```python
from build123d import *

# Parameters (mm, degrees)
EXTRUDE_1_DEPTH     = 15
SKETCH_2_R          = 1.25
CUT_EXTRUDE_1_DEPTH = 30.154759474
SKETCH_3_R          = 1.25
CUT_EXTRUDE_2_DEPTH = 30.154759474
SKETCH_4_R          = 1.5
CUT_EXTRUDE_3_DEPTH = 18
SKETCH_5_W          = 25
SKETCH_5_H          = 15
CUT_EXTRUDE_4_DEPTH = 1
SKETCH_6_W          = 25
SKETCH_6_H          = 15
CUT_EXTRUDE_5_DEPTH = 1


with BuildPart() as part:
    # 草图1 → 凸台-拉伸1 (new body)
    with BuildSketch(Plane(origin=(0, 0, 0), x_dir=(1, 0, 0), z_dir=(0, 1, 0))):
        Polygon((0, 0), (-5, 0), (-5, -15), (20, -15), (20, 0), (15, 0), (15, -11), (0, -11), align=None)
    extrude(amount=EXTRUDE_1_DEPTH)

    # 草图2 → 切除-拉伸1 (cut, through all)
    with BuildSketch(Plane(origin=(0, 0, 0), x_dir=(-1, 0, 0), z_dir=(0, 0, -1))):
        with Locations((-17.5, 4)):
            Circle(SKETCH_2_R)
        with Locations((-17.5, 11)):
            Circle(SKETCH_2_R)
    extrude(amount=-CUT_EXTRUDE_1_DEPTH, mode=Mode.SUBTRACT)

    # 草图3 → 切除-拉伸2 (cut, through all)
    with BuildSketch(Plane(origin=(0, 0, 0), x_dir=(-1, 0, 0), z_dir=(0, 0, -1))):
        with Locations((2.5, 4)):
            Circle(SKETCH_3_R)
        with Locations((2.5, 11)):
            Circle(SKETCH_3_R)
    extrude(amount=-CUT_EXTRUDE_2_DEPTH, mode=Mode.SUBTRACT)

    # 草图4 → 切除-拉伸3 (cut)
    with BuildSketch(Plane.XY.offset(15)):
        with Locations((7.5, 7.5)):
            Circle(SKETCH_4_R)
    extrude(amount=-CUT_EXTRUDE_3_DEPTH, mode=Mode.SUBTRACT)

    # 草图5 → 切除-拉伸4 (cut)
    with BuildSketch(Plane(origin=(0, 0, 0), x_dir=(-1, 0, 0), z_dir=(0, 0, -1))):
        with Locations((-7.5, 7.5)):
            Rectangle(SKETCH_5_W, SKETCH_5_H)
    extrude(amount=-CUT_EXTRUDE_4_DEPTH, mode=Mode.SUBTRACT)

    # 草图6 → 切除-拉伸5 (cut)
    with BuildSketch(Plane.XY.offset(15)):
        with Locations((7.5, 7.5)):
            Rectangle(SKETCH_6_W, SKETCH_6_H)
    extrude(amount=-CUT_EXTRUDE_5_DEPTH, mode=Mode.SUBTRACT)


solid = part.part
```
CAD build for the part. Positions are in the model's coordinates, mm. A direction names the side the tool comes from. Round coordinates to 2 decimals unless told otherwise and drop trailing zeros. Order: outer loops, then holes, each group sorted by start corner. A loop starts at its lowest first (then second) coordinate and runs counter-clockwise, first axis right, second up. Notation, with made-up numbers: (85, -32) - (133, -32) arc R21 ccw to (133, -22) - close; hole circle Ø5 at (57.5, -21.5). An arc over 180 degrees is marked (long way). Use CSV: the item, a comma, the result in double quotes. Start each with the question number.
1) Wall check: L1, parallel to X at y = 5.5, z = 10.5; L2, parallel to Y at x = 16.5, z = 12.5; L3, parallel to Y at x = -2.5, z = 4.25. Give the ranges that are in metal, low to high. Write a range as [from, to].
2) Saw through at B-B (y = 7.5). List the corners of the cut face in (x, z), and give its area (3 significant figures).
3) Two-plate mould, pull along X, no slides. Class faces 3 (the flat face through (0, 7, 6)), 4 (the flat face through (20, 7, 8)), 5 (the cylindrical face through (16.345, 3.521, 7.409)), 6 (the flat face through (-2, 8, 1)): pulls with the +X half, pulls with the -X half, needs draft (parallel to the pull), parting line crosses it, or undercut.
4) Pin check, flat tip, straight feed: pin 1 Ø2 at (x, y) = (17.5, 4) entering from +Z. Stop position of the tip, or through.
5) Saw through at C-C (x = 7.5). List the corners of the cut face in (y, z), and give its area (3 significant figures).
6) Saw through at A-A (z = 3.5). List the corners of the cut face in (x, y), and give its area (3 significant figures).
7) Saw through at D-D (y = 4). List the corners of the cut face in (x, z).
8) Tool access for faces 1 (the cylindrical face through (16.828, 12.054, 7.409)), 2 (the flat face through (9.3, 7.4, 11)): list every direction of +Z, -Z, +X, -X, +Y, -Y with a clear straight run to the whole face (end or side of a thin tool).
Values follow:
1,L1,"x = [-5, 0], [15, 20]"
1,L2,"y = [0, 3.25], [4.75, 10.25], [11.75, 15]"
1,L3,"y = [0, 2.75], [5.25, 9.75], [12.25, 15]"
2,outline,"(-5, 1) - (0, 1) - (0, 11) - (6, 11) - (6, 14) - (-5, 14) - close; (9, 11) - (15, 11) - (15, 1) - (20, 1) - (20, 14) - (9, 14) - close"
2,area,"166 mm2"
3,face 3,"undercut"
3,face 4,"pulls with the +X half"
3,face 5,"undercut"
3,face 6,"needs draft"
4,pin 1,"passes through"
5,outline,"(0, 11) - (6, 11) - (6, 14) - (0, 14) - close; (9, 11) - (15, 11) - (15, 14) - (9, 14) - close"
5,area,"36.0 mm2"
6,outline,"(-5, 0) - (0, 0) - (0, 15) - (-5, 15) - close; (15, 0) - (20, 0) - (20, 15) - (15, 15) - close; hole circle Ø2.5 at (-2.5, 4); hole circle Ø2.5 at (-2.5, 11); hole circle Ø2.5 at (17.5, 4); hole circle Ø2.5 at (17.5, 11)"
6,area,"130 mm2"
7,outline,"(-5, 1) - (-3.75, 1) - (-3.75, 14) - (-5, 14) - close; (-1.25, 1) - (0, 1) - (0, 11) - (15, 11) - (15, 1) - (16.25, 1) - (16.25, 14) - (-1.25, 14) - close; (18.75, 1) - (20, 1) - (20, 14) - (18.75, 14) - close"
8,face 1,"+Z, -Z"
8,face 2,"-Z, +Y, -Y"
